from build123d import *

# Parameters (mm, degrees)
SKETCH1_R           = 1.1
BOSS_EXTRUDE1_DEPTH = 5
BOSS_EXTRUDE2_DEPTH = 9
FILLET1_R           = 15
SKETCH3_R           = 1
CUT_EXTRUDE1_DEPTH  = 16
FILLET2_R           = 3
SKETCH4_R           = 1.9
CUT_EXTRUDE2_DEPTH  = 1
FILLET3_R           = 1.5
FILLET4_R           = 0.5
SKETCH5_W           = 82.891813234
SKETCH5_H           = 4.5
CUT_EXTRUDE3_DEPTH  = 5
SKETCH6_R           = 1
CUT_EXTRUDE4_DEPTH  = 4.5
LPATTERN1_COUNT     = 11
LPATTERN1_PITCH     = 7
FILLET5_R           = 5
FILLET6_R           = 15
SKETCH7_W           = 12
SKETCH7_H           = 5
CUT_EXTRUDE5_DEPTH  = 5
FILLET7_R           = 0.5


with BuildPart() as part:
    # Sketch1 → Boss-Extrude1 (new body)
    with BuildSketch(Plane.XY):
        with BuildLine():
            ThreePointArc((0, 4.5), (-4.5, 0), (0, -4.5))
            Line((0, -4.5), (90, -4.5))
            Line((90, -4.5), (90, 4.5))
            Line((90, 4.5), (0, 4.5))
        make_face()
        Circle(SKETCH1_R, mode=Mode.SUBTRACT)
    extrude(amount=BOSS_EXTRUDE1_DEPTH)

    # Sketch2 → Boss-Extrude2 (add)
    with BuildSketch(Plane(origin=(0, 4.5, 0), x_dir=(1, 0, 0), z_dir=(0, 1, 0))):
        Polygon((90.5, 2), (100, 2), (100, 5.5), (90, 5.5), (90, 0), (90, -5), (90, -10.5), (100, -10.5), (100, -7), (90.5, -7), align=None)
    extrude(amount=-BOSS_EXTRUDE2_DEPTH)

    # Fillet1
    # the kernel refuses this fillet: 15 mm, written as the material it adds along each edge
    with BuildSketch(Plane(origin=(90, -4.5, 0), x_dir=(0, 0, -1), z_dir=(0, 1, 0))) as fillet1_piece_1:
        with BuildLine():
            CenterArc((15, 11.608186766), FILLET1_R, 180, 50.703519761)
            Line((0, 11.608186766), (-0.3, 11.608186766))
            Line((-0.3, 11.608186766), (-0.3, 0))
            Line((-0.3, 0), (0, -0.3))
            ThreePointArc((0, -0.3), (2.75, -0.3), (5.31, -0.232163735))
            Line((5.31, -0.232163735), (5.5, 0))
        make_face()
    extrude(amount=9)
    with BuildSketch(Plane(origin=(90, -4.5, 5), x_dir=(0, 0, 1), z_dir=(0, 1, 0))) as fillet1_piece_2:
        with BuildLine():
            CenterArc((15, -11.608186766), FILLET1_R, 129.296480239, 50.703519761)
            Line((0, -11.608186766), (-0.3, -11.608186766))
            Line((-0.3, -11.608186766), (-0.3, 0))
            Line((-0.3, 0), (0, 0.3))
            ThreePointArc((0, 0.3), (2.75, 0.3), (5.31, 0.232163735))
            Line((5.31, 0.232163735), (5.5, 0))
        make_face()
    extrude(amount=9)

    # Sketch3 → Cut-Extrude1 (cut)
    with BuildSketch(Plane.XY.offset(10.5)):
        with Locations((96, 0)):
            Circle(SKETCH3_R)
    extrude(amount=-CUT_EXTRUDE1_DEPTH, mode=Mode.SUBTRACT)

    # Fillet2
    fillet2_edges = [part.edges().sort_by_distance(p)[0] for p in [
        (100, 4.5, 8.75),
        (100, 4.5, -3.75),
        (100, -4.5, 8.75),
        (100, -4.5, -3.75),
    ]]
    fillet(fillet2_edges, radius=FILLET2_R)

    # Sketch4 → Cut-Extrude2 (cut)
    with BuildSketch(Plane.XY.offset(10.5)):
        with Locations((96, 0)):
            Circle(SKETCH4_R)
    extrude(amount=-CUT_EXTRUDE2_DEPTH, mode=Mode.SUBTRACT)

    # Fillet3
    fillet3_edges = [part.edges().sort_by_distance(p)[0] for p in [
        (90.5, 0, 7),
        (90.5, 0, -2),
    ]]
    fillet(fillet3_edges, radius=FILLET3_R)

    # Fillet4
    fillet4_edges = [part.edges().sort_by_distance(p)[0] for p in [
        (95, 0, -2),
    ]]
    fillet(fillet4_edges, radius=FILLET4_R)

    # Sketch5 → Cut-Extrude3 (cut)
    with BuildSketch(Plane.XY.offset(5)):
        with Locations((36.945906617, 2.25)):
            Rectangle(SKETCH5_W, SKETCH5_H)
    extrude(amount=-CUT_EXTRUDE3_DEPTH, mode=Mode.SUBTRACT)

    # Sketch6 → Cut-Extrude4 (cut)
    with BuildSketch(Plane(origin=(0, 0, 0), x_dir=(1, 0, 0), z_dir=(0, 1, 0))):
        with Locations(Location((74.391813234, -2.5, 0), (0, 0, 270))):
            Circle(SKETCH6_R)
    cut_extrude4 = extrude(amount=-CUT_EXTRUDE4_DEPTH, mode=Mode.SUBTRACT)

    # LPattern1: Cut-Extrude4 ×11
    with Locations(*[(-i * LPATTERN1_PITCH, 0, 0) for i in range(1, LPATTERN1_COUNT)]):
        add(cut_extrude4, mode=Mode.SUBTRACT)

    # Fillet5
    # the kernel refuses this fillet: 5 mm, written as the material it adds along each edge
    with BuildSketch(Plane(origin=(78.391813234, 0, 5), x_dir=(0, 1, 0), z_dir=(0, 0, -1))) as fillet5_piece_1_section:
        with BuildLine():
            CenterArc((5, -4.974937186), FILLET5_R, 95.739170477, 84.260829523)
            Line((0, -4.974937186), (0, 0))
            Line((0, 0), (4.5, 0))
        make_face()
    fillet5_piece_1 = extrude(amount=5, mode=Mode.PRIVATE)
    fillet5_piece_1 = fillet5_piece_1 - Plane(origin=(74.391813234, 1.284484558, 2.5), x_dir=(0, 0, 1), z_dir=(0, 1, 0)) * Cylinder(1, 30, mode=Mode.PRIVATE)
    add(fillet5_piece_1)

    # Fillet6
    fillet6_edges = [part.edges().sort_by_distance(p)[0] for p in [
        (78.391813234, 4.5, 2.5),
    ]]
    fillet(fillet6_edges, radius=FILLET6_R)

    # Sketch7 → Cut-Extrude5 (cut)
    with BuildSketch(Plane(origin=(0, 0, 0), x_dir=(1, 0, 0), z_dir=(0, 1, 0))):
        with Locations((1.5, -2.5)):
            Rectangle(SKETCH7_W, SKETCH7_H)
    extrude(amount=-CUT_EXTRUDE5_DEPTH, mode=Mode.SUBTRACT)

    # Fillet7
    fillet7_edges = [part.edges().sort_by_distance(p)[0] for p in [
        (95, 0, 7),
        (95, 0, -5.5),
    ]]
    fillet(fillet7_edges, radius=FILLET7_R)


solid = part.part
Check sheet for the modelled part. Datum: model origin and axes. Units: mm. A direction names the side the tool comes from. Round coordinates to 2 decimals unless told otherwise and drop trailing zeros. Order: outer loops, then holes, each group sorted by start corner. A loop starts at its lowest first (then second) coordinate and runs counter-clockwise, first axis right, second up. Notation, with made-up numbers: M 20.25,52.5 L 75.25,52.5 A12 ccw 75.25,66.5 Z; hole C 10.25,29 d10. An arc over 180 degrees is marked long. One line per item, written item: value. Start each with the question number.
1. Access from +Z, -Z, +X, -X, +Y, -Y to the whole of each face (thin tool, end or side, straight path). Record for faces 1 (the flat face through (97, -1, 9.5)), 2 (the flat face through (43, -2, 5)), 3 (the flat face through (43, -2, 0)), 4 (the flat face through (94, 0, 7)).
2. Release check for a two-part mould opening along X. For faces 5 (the cylindrical face through (75.81, 0.61, 2.54)), 6 (the cylindrical face through (26.383, -2.218, 2.37)), 7 (the cylindrical face through (99.1, 3.64, -3.77)) record: released by +X, released by -X, zero draft, split by the parting line, or undercut.
3. Section check A-A on x = 96. Enter the section's corners in (y, z).
4. Scan lines: line 1 along Z through (x, y) = (39.5, -3.75); line 2 along Y through (x, z) = (72.5, 4); line 3 along Z through (x, y) = (64, -3.5). Record each from-to range of solid material in increasing order.
5. Gauge pin test, flat ends, axial feed: P1, Ø3, axis at y = -1, z = -1, coming from the -X side; P2, Ø2.5, axis at x = 60.39, z = 2.5, coming from the +Y side; P3, Ø1, axis at x = 60.5, y = -0.5, coming from the +Z side; P4, Ø4, axis at y = 2.5, z = 5, coming from the -X side. Record the tip position at first contact, or that the pin passes through.
6. Section check B-B on y = -3.5. Give the number of separate pieces and of enclosed holes in the cut face, and give its area (3 significant figures).
7. Section check C-C on x = 22. Enter the section's corners in (y, z), and give its area (3 significant figures).
Results found:
1. face 1: +Z
1. face 2: +Z, -X, +Y, -Y
1. face 3: -Z, -X, +Y, -Y
1. face 4: +X, +Y, -Y
2. face 5: released by -X
2. face 6: undercut
2. face 7: released by +X
3. outline: M -4.5,-5.5 L -1.5,-5.5 A0.5 ccw -1,-5 L -1,-2.5 A0.5 ccw -1.5,-2 L -4.5,-2 Z; M -4.5,7 L -1.5,7 A0.5 ccw -1,7.5 L -1,9.5 L -1.9,9.5 L -1.9,10.5 L -4.5,10.5 Z; M 1,-5 A0.5 ccw 1.5,-5.5 L 4.5,-5.5 L 4.5,-2 L 1.5,-2 A0.5 ccw 1,-2.5 Z; M 1,7.5 A0.5 ccw 1.5,7 L 4.5,7 L 4.5,10.5 L 1.9,10.5 L 1.9,9.5 L 1,9.5 Z
4. line 1: 0 to 1.51, 3.49 to 5
4. line 2: -4.5 to 0
4. line 3: 0 to 5
5. P1: x = 7.5
5. P2: y = 0
5. P3: z = 5
5. P4: x = 75.6
6. separate pieces: 1
6. enclosed holes: 10
6. area: 490 mm^2
7. outline: M -4.5,0 L 0,0 L 0,5 L -4.5,5 Z
7. area: 22.5 mm^2
